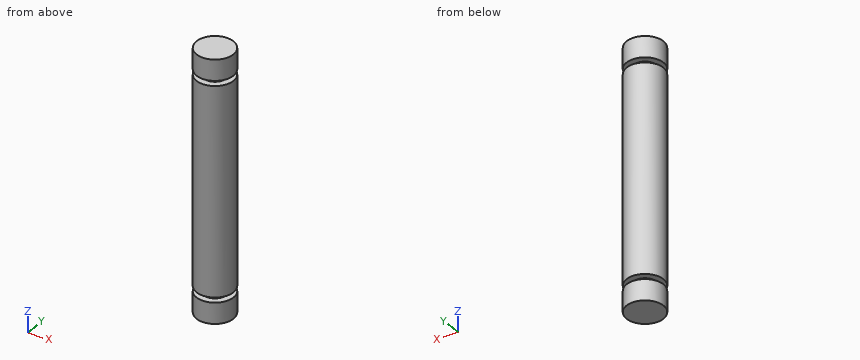
```python
from build123d import *

# Parameters (mm, degrees)
SKETCH1_R           = 2.5
BOSS_EXTRUDE1_DEPTH = 35
SKETCH2_W           = 0.68
SKETCH2_H           = 0.9


with BuildPart() as part:
    # Sketch1 → Boss-Extrude1 (new body)
    with BuildSketch(Plane.XY):
        Circle(SKETCH1_R)
    extrude(amount=BOSS_EXTRUDE1_DEPTH)

    # Sketch2 → Cut-Revolve1 (revolve, cut)
    with BuildSketch(Plane(origin=(0, 0, 0), x_dir=(0, 0, -1), z_dir=(1, 0, 0))):
        with Locations((-31.84, 2.05)):
            Rectangle(SKETCH2_W, SKETCH2_H)
        with Locations((-3.16, 2.05)):
            Rectangle(SKETCH2_W, SKETCH2_H)
    revolve(axis=Axis((0, 0, 35), (0, 0, -1)), mode=Mode.SUBTRACT)


solid = part.part
```
The listing builds one solid part. Answer for the finished solid, in the listing's coordinates (mm). Coordinates: 2 decimals unless noted, no trailing zeros. Write each loop counter-clockwise with the first axis right and the second up, starting at its lowest first coordinate (ties: lowest second). Pieces come first, ordered by that corner, then holes. Notation, with made-up numbers: (-18, -24) - (24, -24) arc R28 cw to (24, 1) - close; hole circle Ø1 at (18.5, 89). An arc over 180 degrees is marked (long way). Return JSON: item names as keys, results as strings. Group by question number.
1. A cutting plane is placed at C-C, the plane x = -0.3. Determine the outline of the cut face in (y, z), plus the area to 3 significant figures.
2. A cutting plane is placed at A-A, the plane x = -2.2. Determine the outline of the cut face in (y, z).
3. A cutting plane is placed at B-B, the plane y = -0.7. Determine the outline of the cut face in (x, z), plus the area to 3 significant figures.
4. Given pin 1 (1 mm diameter, centred on y = 1, z = 12, fed in from +X), flat-ended and moving along its own axis, determine where the tip first touches the part or whether it passes through.
5. Straight lines are drawn through the part: L1, parallel to Z at x = 1.3, y = 1; L2, parallel to X at y = 0.1, z = 17.5; L3, parallel to Y at x = 0.5, z = 11. For each, find the intervals that lie inside material, in ascending order.
Ans:
{
 "1": {"outline": "(-2.48, 0) - (2.48, 0) - (2.48, 2.82) - (1.57, 2.82) - (1.57, 3.5) - (2.48, 3.5) - (2.48, 31.5) - (1.57, 31.5) - (1.57, 32.18) - (2.48, 32.18) - (2.48, 35) - (-2.48, 35) - (-2.48, 32.18) - (-1.57, 32.18) - (-1.57, 31.5) - (-2.48, 31.5) - (-2.48, 3.5) - (-1.57, 3.5) - (-1.57, 2.82) - (-2.48, 2.82) - close", "area": "171 mm²"},
 "2": {"outline": "(-1.19, 0) - (1.19, 0) - (1.19, 2.82) - (-1.19, 2.82) - close; (-1.19, 3.5) - (1.19, 3.5) - (1.19, 31.5) - (-1.19, 31.5) - close; (-1.19, 32.18) - (1.19, 32.18) - (1.19, 35) - (-1.19, 35) - close"},
 "3": {"outline": "(-2.4, 0) - (2.4, 0) - (2.4, 2.82) - (1.44, 2.82) - (1.44, 3.5) - (2.4, 3.5) - (2.4, 31.5) - (1.44, 31.5) - (1.44, 32.18) - (2.4, 32.18) - (2.4, 35) - (-2.4, 35) - (-2.4, 32.18) - (-1.44, 32.18) - (-1.44, 31.5) - (-2.4, 31.5) - (-2.4, 3.5) - (-1.44, 3.5) - (-1.44, 2.82) - (-2.4, 2.82) - close", "area": "165 mm²"},
 "4": {"pin 1": "x = 2.45"},
 "5": {"L1": "0 to 2.82, 3.5 to 31.5, 32.18 to 35", "L2": "-2.5 to 2.5", "L3": "-2.45 to 2.45"}
}
